```python
from build123d import *

# Parameters (mm, degrees)
F0_R     = 10
F1_DEPTH = 15


# Not quite as in the source:
# - a feature names something its author has since deleted; it is built from what else it names


with BuildPart() as f1:
    # F0 (on Front) → F1 (new body)
    with BuildSketch(Plane.XZ):
        with BuildLine():
            ThreePointArc((-12.4862537895, 224.2308067578), (0.2931105859, 212.3203037661), (12.5, 224.8168667409))
            ThreePointArc((12.5, 224.8168667409), (0.293876674, 237.3134117235), (-12.4861818401, 225.404457633))
            Line((-12.4861818401, 225.404457633), (-12.4862537895, 224.2308067578))
        make_face()
        with Locations((0, 224.8168667409)):
            Circle(F0_R, mode=Mode.SUBTRACT)
        with BuildLine():
            Line((12.5, 15.3332800892), (12.5, 224.8168667409))
            ThreePointArc((12.5, 224.8168667409), (0.2931105859, 212.3203037661), (-12.4862537895, 224.2308067578))
            Line((-12.4862537895, 224.2308067578), (-12.4990556694, 15.4044580276))
            ThreePointArc((-12.4990556694, 15.4044580276), (-15.36849483, 8.3940010786), (-22.3294631759, 5.4065092509))
            Line((-22.3294631759, 5.4065092509), (-22.5, -7))
            ThreePointArc((-22.5, -7), (-19.5710678119, -14.0710678119), (-12.5, -17))
            Line((-12.5, -17), (12.5, -17))
            ThreePointArc((12.5, -17), (19.5710678119, -14.0710678119), (22.5, -7))
            Line((22.5, -7), (22.3300547766, 5.3347242624))
            ThreePointArc((22.3300547766, 5.3347242624), (15.3691006095, 8.3225544574), (12.5, 15.3332800892))
        make_face()
        with BuildLine():
            ThreePointArc((-12.4999999765, 0.0007662994), (0.0003831497, 12.4999999941), (12.5, 0))
            ThreePointArc((12.5, 0), (0, -12.5), (-12.5, 0))
            Line((-12.5000000235, 0), (-12.4999999765, 0.0007662994))
        make_face(mode=Mode.SUBTRACT)
    extrude(amount=F1_DEPTH)


solid = f1.part
```
Verification items for the finished model (mm, model axes). A direction names the side the tool comes from. Coordinates: 2 decimals unless noted, no trailing zeros. Write each loop counter-clockwise with the first axis right and the second up, starting at its lowest first coordinate (ties: lowest second). Pieces come first, ordered by that corner, then holes. Notation, with made-up numbers: (51.5, 54.5) - (57.5, 54.5) arc R23 ccw to (57.5, 84.5) - close; hole circle Ø4 at (59.5, -15.5). An arc over 180 degrees is marked (long way). Write item = value, one per line.
Q1. Cross-section at A-A (x = 0). Enter the section's corners in (y, z), plus the area to 3 significant figures.
Answer:
outline = (-15, -17) - (0, -17) - (0, -12.5) - (-15, -12.5) - close; (-15, 12.5) - (0, 12.5) - (0, 214.82) - (-15, 214.82) - close; (-15, 234.82) - (0, 234.82) - (0, 237.32) - (-15, 237.32) - close
area = 3,140 mm²
Q2. Cross-section at C-C (z = 66.5). Enter the section's corners in (x, y).
Answer:
outline = (-12.5, -15) - (12.5, -15) - (12.5, 0) - (-12.5, 0) - close
Q3. Cross-section at D-D (z = 182). Enter the section's corners in (x, y).
Answer:
outline = (-12.49, -15) - (12.5, -15) - (12.5, 0) - (-12.49, 0) - close
Q4. Go/stop test with flat-tipped pins: pin 1 Ø0.6 at (y, z) = (-7.5, 225) entering from -X; pin 2 Ø4 at (x, z) = (15, 171) entering from +Y; pin 3 Ø4 at (x, y) = (-7.5, -10) entering from +Z; pin 4 Ø8 at (y, z) = (-8, 58) entering from +X. Record where each tip stops, or that it passes through.
Answer:
pin_1 = -12.49
pin_2 = through
pin_3 = 236.04
pin_4 = 12.5
Q5. Material ranges on L1, parallel to Z at x = 0, y = -8; L2, parallel to X at y = -4.5, z = 68; L3, parallel to X at y = -13, z = 5, recorded low to high. Write a range as from..to.
Answer:
L1 = -17..-12.5, 12.5..214.82, 234.82..237.32
L2 = -12.5..12.5
L3 = -22.34..-11.46, 11.46..22.33
Q6. Access from +Z, -Z, +X, -X, +Y, -Y to the whole of each face (thin tool, end or side, straight path). Record for faces 1 (the face through (19.49, -7.4, -14.15)), 2 (the face through (12.5, -7, 119)).
Answer:
face_1 = -Z, +X, +Y, -Y
face_2 = +Z, +X, +Y, -Y
Q7. Cross-section at B-B (y = -4.5). Give the number of separate pieces and of enclosed holes in the cut face, plus the area to 3 significant figures.
Answer:
separate_pieces = 1
enclosed_holes = 2
area = 5,930 mm²
Q8. Mould release check, pull along Z, two halves, no side actions. Record for faces 3 (the face through (15.446, -7.395, 8.245)), 4 (the face through (-1.3, -7.4, 234.73)), 5 (the face through (0, 0, 112)): released by +Z, released by -Z, zero draft, split by the parting line, or undercut.
Answer:
face_3 = released by +Z
face_4 = undercut
face_5 = zero draft
